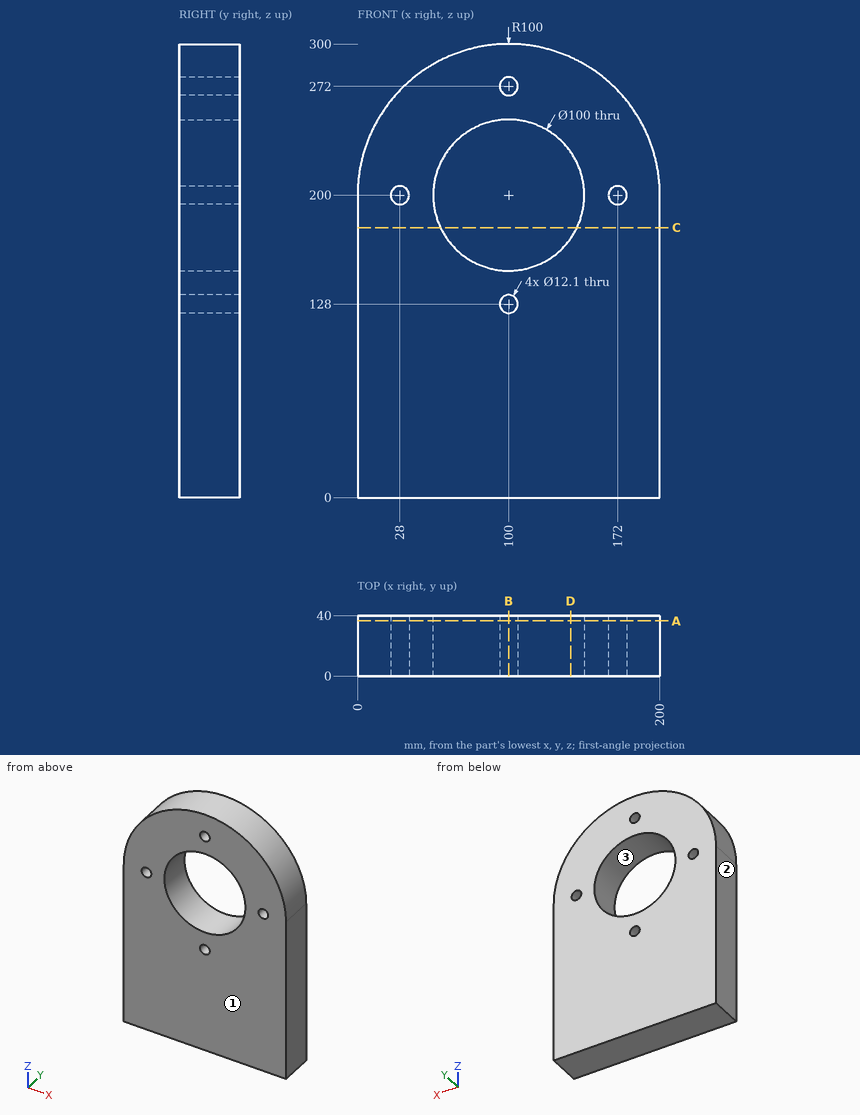
Part print with two shaded views. Sizes in mm from the minimum x, y, z corner. Round coordinates to 2 decimals unless told otherwise and drop trailing zeros. Write each loop counter-clockwise with the first axis right and the second up, starting at its lowest first coordinate (ties: lowest second). Pieces come first, ordered by that corner, then holes. Notation, with made-up numbers: M 84.5,-9.75 L 94.5,-9.75 A31 ccw 94.5,22.25 Z; hole C 49,-13.5 d10. An arc over 180 degrees is marked long. Put each result on its own line as item: value. Start each with the question number.
1) Saw through at B-B, the plane x = 100. Write the cut outline in (y, z), and give its area (3 significant figures).
2) Drill centre lines: probe 1 along Z at (x, y) = (100, 24); probe 2 along X at (y, z) = (37, 200.5); probe 3 along X at (y, z) = (16, 128). Where is each one in solid material? Low to high. Write a range as [from, to].
3) Saw through at A-A, the plane y = 36.5. Write the cut outline in (x, z), and give its area (3 significant figures).
4) Saw through at D-D, the plane x = 141. Write the cut outline in (y, z), and give its area (3 significant figures).
5) Saw through at C-C, the plane z = 178.5. Write the cut outline in (x, y).
6) Pin check, flat tips, straight feed: pin 1 Ø10 at (x, y) = (64, 31.5) entering from +Z; pin 2 Ø12 at (x, z) = (117.5, 47) entering from -Y; pin 3 Ø6 at (x, y) = (139.5, 18) entering from +Z; pin 4 Ø1 at (y, z) = (24.5, 236) entering from -X. Stop position of each tip, or through.
7) Pull direction X, two halves, no side cores. Call the marked faces 1, 2 and 3: pulls with the +X half, pulls with the -X half, needs draft (parallel to the pull), parting line crosses it, or undercut.
Resolved:
1. outline: M 0,0 L 40,0 L 40,121.95 L 0,121.95 Z; M 0,134.05 L 40,134.05 L 40,150 L 0,150 Z; M 0,250 L 40,250 L 40,265.95 L 0,265.95 Z; M 0,278.05 L 40,278.05 L 40,300 L 0,300 Z
1. area: 7,030 mm²
2. probe 1: [0, 121.95], [134.05, 150], [250, 265.95], [278.05, 300]
2. probe 2: [0, 21.97], [34.03, 50], [150, 165.97], [178.03, 200]
2. probe 3: [0, 93.95], [106.05, 200]
3. outline: M 0,0 L 200,0 L 200,200 A100 ccw 0,200 Z; hole C 28,200 d12.1; hole C 100,200 d100; hole C 100,128 d12.1; hole C 100,272 d12.1; hole C 172,200 d12.1
3. area: 47,400 mm²
4. outline: M 0,0 L 40,0 L 40,171.38 L 0,171.38 Z; M 0,228.62 L 40,228.62 L 40,291.21 L 0,291.21 Z
4. area: 9,360 mm²
5. outline: M 0,0 L 54.86,0 L 54.86,40 L 0,40 Z; M 145.14,0 L 200,0 L 200,40 L 145.14,40 Z
6. pin 1: z = 295.07
6. pin 2: y = 0
6. pin 3: z = 293.1
6. pin 4: x = 6.51
7. face 1: needs draft
7. face 2: pulls with the -X half
7. face 3: undercut
